Can you work these out from the model? Positions are in its coordinate system, mm. Coordinates: 2 decimals unless noted, no trailing zeros. Order: outer loops, then holes, each group sorted by start corner. A loop starts at its lowest first (then second) coordinate and runs counter-clockwise, first axis right, second up. Notation, with made-up numbers: (-12, 75.5) -> (43, 75.5) arc R24 cw to (43, 97.5) -> close; hole circle Ø4 at (31.25, -31.75). An arc over 180 degrees is marked (long way). Answer as a JSON object with one key per item and string values. Group by question number.
(1) If we mould it in two halves opening along X, with no side actions, what happens to faces 1 (the cylindrical face through (51.51, -55.37, 1.97)), 2 (the flat face through (-1, 1, 4)), 3 (the cylindrical face through (-68.49, 54.63, 1.97)), 4 (the cylindrical face through (-78.289, -68.196, 2.028))? For each: pulls with the +X half, pulls with the -X half, needs draft (parallel to the pull), parting line crosses it, or undercut.
(2) I want a section at C-C, the plane z = 2.15. List the corners of the cut face in (x, y) for me, plus the area to 3 significant figures.
(3) I want a section at B-B, the plane x = 60. List the corners of the cut face in (y, z) for me, plus the area to 3 significant figures.
(4) I need wall thicknesses on line 1 (Y direction, x = 60, z = 1.6); line 2 (Y direction, x = -55, z = 0.8); line 3 (X direction, y = 61.5, z = 0.9). Which ranges of each line are inside material? Lowest first, please.
(5) I want a section at A-A, the plane y = 55. List the corners of the cut face in (x, z) for me, plus the area to 3 significant figures.
Autodesk Inventor part; units mm, degrees
ref_plane "YZ Plane" through (0, 0, 0) normal (1, 0, 0) x (0, 1, 0)
ref_plane "XZ Plane" through (0, 0, 0) normal (0, 1, 0) x (-1, 0, 0)
ref_plane "XY Plane" through (0, 0, 0) normal (0, 0, 1) x (1, 0, 0)
sketch3d "3D Sketch1"
sketch "Sketch1" plane through (0, 0, 0) normal (0, 0, 1) x (1, 0, 0)
  line L0 (-56, 70) -> (56, 70)
  line L1 (56, 70) -> (56, -70) construction
  line L2 (56, -70) -> (-56, -70)
  line L3 (-56, -70) -> (-56, 70) construction
  line L4 (-56, 70) -> (56, -70) construction
  line L5 (56, 70) -> (-56, -70) construction
  line L6 (56, -70) -> (80, -70)
  line L7 (80, -70) -> (80, 70)
  line L8 (80, 70) -> (56, 70)
  line L9 (-56, -70) -> (-80, -70)
  line L10 (-80, -70) -> (-80, 70)
  line L11 (-80, 70) -> (-56, 70)
  circle A0 centre (60, -55) radius 8.5
  circle A1 centre (60, 55) radius 8.5
  circle A2 centre (-60, -55) radius 8.5
  circle A3 centre (-60, 55) radius 8.5
  line L12 (0, -70) -> (0, 70) construction
  line L13 (80, 0) -> (-80, 0) construction
  point P0 (0, 0)
  dimension "d30" = 140
  dimension "d34" = 160
  dimension "d35" = 17
  dimension "d36" = 20
  dimension "d37" = 15
extrude "Plate1" add sketch "Sketch1" along normal blind 4
fillet "Corner Round1" radius 6 4 edges at (80, 70, 2) (-80, 70, 2) (-80, -70, 2) (80, -70, 2)
equation "\"d6\" = Thickness"
equation "\"BendReliefWidth\" = Thickness"
equation "\"BendReliefDepth\" = 0.5 * Thickness"
equation "\"CornerReliefSize\" = 4 * Thickness"
equation "\"MinimumRemnant\" = 2 * Thickness"
equation "\"TransitionRadius\" = BendRadius"
equation "\"JacobiRadiusSize\" = BendRadius"
equation "\"GapSize\" = Thickness"
properties part number "ASY MSC 909 base frame transverse" material "Steel"
Computed values:
{
 "1": {"face 1": "undercut", "face 2": "needs draft", "face 3": "undercut", "face 4": "pulls with the -X half"},
 "2": {"outline": "(-80, -64) arc R6 ccw to (-74, -70) -> (74, -70) arc R6 ccw to (80, -64) -> (80, 64) arc R6 ccw to (74, 70) -> (-74, 70) arc R6 ccw to (-80, 64) -> close; hole circle Ø17 at (-60, -55); hole circle Ø17 at (-60, 55); hole circle Ø17 at (60, -55); hole circle Ø17 at (60, 55)", "area": "21,500 mm2"},
 "3": {"outline": "(-70, 0) -> (-63.5, 0) -> (-63.5, 4) -> (-70, 4) -> close; (-46.5, 0) -> (46.5, 0) -> (46.5, 4) -> (-46.5, 4) -> close; (63.5, 0) -> (70, 0) -> (70, 4) -> (63.5, 4) -> close", "area": "424 mm2"},
 "4": {"line 1": "y = -70 to -63.5, -46.5 to 46.5, 63.5 to 70", "line 2": "y = -70 to -61.87, -48.13 to 48.13, 61.87 to 70", "line 3": "x = -80 to -65.48, -54.52 to 54.52, 65.48 to 80"},
 "5": {"outline": "(-80, 0) -> (-68.5, 0) -> (-68.5, 4) -> (-80, 4) -> close; (-51.5, 0) -> (51.5, 0) -> (51.5, 4) -> (-51.5, 4) -> close; (68.5, 0) -> (80, 0) -> (80, 4) -> (68.5, 4) -> close", "area": "504 mm2"}
}
